The model under review builds one solid part; all positions refer to its coordinate system, in mm. Round coordinates to 2 decimals unless told otherwise and drop trailing zeros. Write each loop counter-clockwise with the first axis right and the second up, starting at its lowest first coordinate (ties: lowest second). Pieces come first, ordered by that corner, then holes.
Item 1: Draft analysis for pull direction Y (two halves, no side actions). For faces 1 (the face through (36, 31, 5.75)), 2 (the face through (-1, -33, 6)), 3 (the face through (-51, 0, 8)), 4 (the face through (-1, 0, 0)), state which applies: +Y half, -Y half, draft (parallel to the pull), parting line (faces both ways), or undercut.
Item 2: To check wall thickness, follow L1, parallel to Y at x = 36, z = 9; L2, parallel to Y at x = 53.5, z = 9; L3, parallel to X at y = -16, z = 11.5. State the ranges of each line that lie inside material, in increasing order.
Item 3: Add section C-C (x = 53.5). Give the boundary of the cut face in (y, z), plus the area to 4 significant figures.
Item 4: Add section B-B (y = -23.5). Give the boundary of the cut face in (x, z), plus the area to 3 significant figures.
Item 5: Clearance check with flat-ended pins moving along their axes: pin 1 Ø2.5 at (x, y) = (53.5, 14) entering from +Z; pin 2 Ø1 at (x, y) = (-19, -15.5) entering from +Z. State where each tip first meets the part, or that it passes through.
Item 6: Add section D-D (x = 23.5). Give the boundary of the cut face in (y, z).
Item 7: Add section A-A (z = 9). State how many separate pieces and enclosed holes the cut face has, plus the area to 3 significant figures.
```python
from build123d import *

# Parameters (mm, degrees)
F0_W     = 112
F0_H     = 66
F1_DEPTH = 12
F2_T     = -5
F3_R     = 1.5
F4_DEPTH = 6.25


with BuildPart() as f1:
    # F0 (on Top) → F1 (new body)
    with BuildSketch(Plane.XY):
        Rectangle(F0_W, F0_H)
    extrude(amount=F1_DEPTH)

    # F2
    f2_openings = [f1.faces().sort_by_distance(p)[0] for p in [
        (0, 0, 12),
    ]]
    offset(amount=F2_T, openings=f2_openings)

    # F3 (on face) → F4 (cut)
    with BuildSketch(Plane.XY.offset(12)):
        with Locations((-53.5, 14)):
            Circle(F3_R)
        with Locations((-53.5, -14)):
            Circle(F3_R)
        with Locations((-36, 30.5)):
            Circle(F3_R)
        with Locations((-15, 30.5)):
            Circle(F3_R)
        with Locations((15, 30.5)):
            Circle(F3_R)
        with Locations((36, 30.5)):
            Circle(F3_R)
        with Locations((53.5, 14)):
            Circle(F3_R)
        with Locations((53.5, -14)):
            Circle(F3_R)
        with Locations((36, -30.5)):
            Circle(F3_R)
        with Locations((15, -30.5)):
            Circle(F3_R)
        with Locations((-15, -30.5)):
            Circle(F3_R)
        with Locations((-36, -30.5)):
            Circle(F3_R)
    extrude(amount=-F4_DEPTH, mode=Mode.SUBTRACT)


solid = f1.part
```
Numbers:
1. face 1: undercut
1. face 2: -Y half
1. face 3: undercut
1. face 4: draft
2. L1: y = -33 to -32, -29 to -28, 28 to 29, 32 to 33
2. L2: y = -33 to -15.5, -12.5 to 12.5, 15.5 to 33
2. L3: x = -56 to -51, 51 to 56
3. outline: (-33, 0) - (33, 0) - (33, 12) - (15.5, 12) - (15.5, 5.75) - (12.5, 5.75) - (12.5, 12) - (-12.5, 12) - (-12.5, 5.75) - (-15.5, 5.75) - (-15.5, 12) - (-33, 12) - close
3. area: 754.5 mm2
4. outline: (-56, 0) - (56, 0) - (56, 12) - (51, 12) - (51, 5) - (-51, 5) - (-51, 12) - (-56, 12) - close
4. area: 630 mm2
5. pin 1: stops at z = 5.75
5. pin 2: stops at z = 5
6. outline: (-33, 0) - (33, 0) - (33, 12) - (28, 12) - (28, 5) - (-28, 5) - (-28, 12) - (-33, 12) - close
7. separate pieces: 1
7. enclosed holes: 13
7. area: 1,600 mm2
